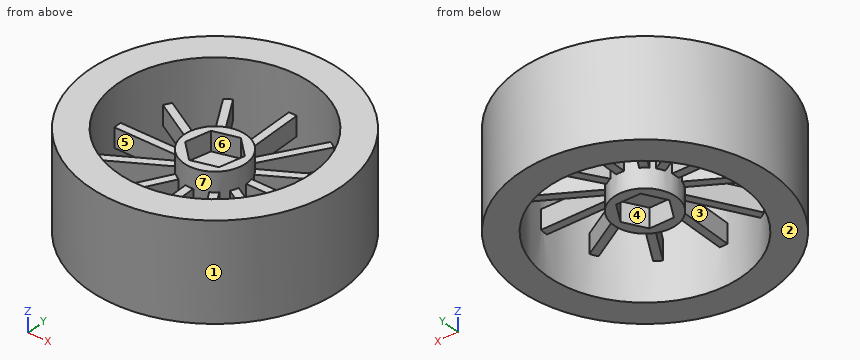
```python
from build123d import *

# Parameters (mm, degrees)
SKETCH_1_R          = 32.5
EXTRUDE_1_DEPTH     = 25
SKETCH_2_R          = 25
CUT_EXTRUDE_1_DEPTH = 25
SKETCH_6_R          = 8
EXTRUDE_3_DEPTH     = 20
SKETCH_7_R          = 8
CUT_EXTRUDE_2_DEPTH = 5
CUT_EXTRUDE_3_DEPTH = 5
CUT_EXTRUDE_4_DEPTH = 5
SKETCH_11_W         = 21
SKETCH_11_H         = 2
EXTRUDE_1_2_DEPTH   = 5
SKETCH_15_W         = 18
SKETCH_15_H         = 2
EXTRUDE_8_DEPTH     = 5
SKETCH_17_W         = 2
SKETCH_17_H         = 19.626417589
EXTRUDE_9_DEPTH     = 5
SKETCH_19_W         = 2
SKETCH_19_H         = 25
EXTRUDE_10_DEPTH    = 5
EXTRUDE_12_DEPTH    = 5
EXTRUDE_13_DEPTH    = 5
EXTRUDE_16_DEPTH    = 5
EXTRUDE_18_DEPTH    = 5
EXTRUDE_20_DEPTH    = 5
EXTRUDE_21_DEPTH    = 5
EXTRUDE_22_DEPTH    = 5
EXTRUDE_23_DEPTH    = 5


with BuildPart() as part:
    # 草图1 → Extrude 1 (new body)
    with BuildSketch(Plane.XY):
        Circle(SKETCH_1_R)
    extrude(amount=EXTRUDE_1_DEPTH)

    # 草图2 → 切除-拉伸1 (cut)
    with BuildSketch(Plane(origin=(0, 0, 0), x_dir=(-1, 0, 0), z_dir=(0, 0, -1))):
        Circle(SKETCH_2_R)
    extrude(amount=-CUT_EXTRUDE_1_DEPTH, mode=Mode.SUBTRACT)



with BuildPart() as body_2:
    # 草图6 → 凸台-拉伸3 (new body)
    with BuildSketch(Plane(origin=(0, 0, 0), x_dir=(-1, 0, 0), z_dir=(0, 0, -1))):
        Circle(SKETCH_6_R)
    extrude(amount=-EXTRUDE_3_DEPTH)

    # 草图7 → 切除-拉伸2 (cut)
    with BuildSketch(Plane(origin=(0, 0, 0), x_dir=(-1, 0, 0), z_dir=(0, 0, -1))):
        Circle(SKETCH_7_R)
    extrude(amount=-CUT_EXTRUDE_2_DEPTH, mode=Mode.SUBTRACT)

    # 草图8 → 切除-拉伸3 (cut)
    with BuildSketch(Plane(origin=(0, 0, 5), x_dir=(-1, 0, 0), z_dir=(0, 0, -1))):
        Polygon((6.204878503, 0), (3.102439251, 5.373582411), (-3.102439251, 5.373582411), (-6.204878503, 0), (-3.102439251, -5.373582411), (3.102439251, -5.373582411), align=None)
    extrude(amount=-CUT_EXTRUDE_3_DEPTH, mode=Mode.SUBTRACT)

    # 草图9 → 切除-拉伸4 (cut)
    with BuildSketch(Plane.XY.offset(20)):
        Polygon((-1.630765345, -6.252377794), (4.599335331, -4.538473114), (6.230100676, 1.713904681), (1.630765345, 6.252377794), (-4.599335331, 4.538473114), (-6.230100676, -1.713904681), align=None)
    extrude(amount=-CUT_EXTRUDE_4_DEPTH, mode=Mode.SUBTRACT)


with BuildPart() as part_1:
    add(part.part)

    add(body_2.part)  # Extrude 1 2 merges body 2
    # 草图11 → Extrude 1 2 (add)
    with BuildSketch(Plane(origin=(0, -0.732123309, 10), x_dir=(-1, 0, 0), z_dir=(0, 0, -1))):
        with Locations((17.554946424, 1)):
            Rectangle(SKETCH_11_W, SKETCH_11_H)
    extrude(amount=-EXTRUDE_1_2_DEPTH)

    # 草图15 → 拉伸-薄壁8 (add)
    with BuildSketch(Plane(origin=(0.783900643, -0.087404702, 10), x_dir=(-1, 0, 0), z_dir=(0, 0, -1))):
        with Locations((-15.204878503, 1)):
            Rectangle(SKETCH_15_W, SKETCH_15_H)
    extrude(amount=-EXTRUDE_8_DEPTH)

    # 草图17 → 拉伸-薄壁9 (add)
    with BuildSketch(Plane(origin=(1.021360023, 0, 10), x_dir=(-1, 0, 0), z_dir=(0, 0, -1))):
        with Locations((1, 15.186791206)):
            Rectangle(SKETCH_17_W, SKETCH_17_H)
    extrude(amount=-EXTRUDE_9_DEPTH)

    # 草图19 → 拉伸-薄壁10 (add)
    with BuildSketch(Plane(origin=(0, 0, 10), x_dir=(-1, 0, 0), z_dir=(0, 0, -1))):
        with Locations((0.222489214, -12.5)):
            Rectangle(SKETCH_19_W, SKETCH_19_H)
    extrude(amount=-EXTRUDE_10_DEPTH)

    # 草图22 → 拉伸-薄壁12 (add)
    with BuildSketch(Plane(origin=(0.523395748, 0, 10), x_dir=(-1, 0, 0), z_dir=(0, 0, -1))):
        Polygon((0, 0), (-13.36975493, 21.124621964), (-11.679785173, 22.194202358), (1.689969757, 1.069580394), align=None)
    extrude(amount=-EXTRUDE_12_DEPTH)

    # 草图23 → 拉伸-薄壁13 (add)
    with BuildSketch(Plane(origin=(0, -0.702264438, 10), x_dir=(-1, 0, 0), z_dir=(0, 0, -1))):
        Polygon((0, 0), (-22.409578035, 12.938175911), (-21.409578035, 14.670226719), (1, 1.732050808), align=None)
    extrude(amount=-EXTRUDE_13_DEPTH)

    # 草图25 → 拉伸-薄壁16 (add)
    with BuildSketch(Plane(origin=(0, 0.899260589, 10), x_dir=(-1, 0, 0), z_dir=(0, 0, -1))):
        Polygon((0, 0), (21.650635095, 12.5), (22.650635095, 10.767949192), (1, -1.732050808), align=None)
    extrude(amount=-EXTRUDE_16_DEPTH)

    # 草图26 → 拉伸-薄壁18 (add)
    with BuildSketch(Plane(origin=(0, 0, 10), x_dir=(-1, 0, 0), z_dir=(0, 0, -1))):
        Polygon((0, 0), (13.491648386, 23.368220483), (15.223699194, 22.368220483), (1.732050808, -1), align=None)
    extrude(amount=-EXTRUDE_18_DEPTH)

    # 草图27 → 拉伸-薄壁20 (add)
    with BuildSketch(Plane(origin=(0, 0, 10), x_dir=(-1, 0, 0), z_dir=(0, 0, -1))):
        Polygon((0, 0), (-23.067411296, -13.317976121), (-24.067411296, -11.585925314), (-1, 1.732050808), align=None)
    extrude(amount=-EXTRUDE_20_DEPTH)

    # 草图28 → 拉伸-薄壁21 (add)
    with BuildSketch(Plane(origin=(0, 0, 10), x_dir=(-1, 0, 0), z_dir=(0, 0, -1))):
        Polygon((0, 0), (-13.731376059, -23.783440992), (-15.463426867, -22.783440992), (-1.732050808, 1), align=None)
    extrude(amount=-EXTRUDE_21_DEPTH)

    # 草图29 → 拉伸-薄壁22 (add)
    with BuildSketch(Plane(origin=(-1.752500167, 0, 10), x_dir=(-1, 0, 0), z_dir=(0, 0, -1))):
        Polygon((0, 0), (13.9695501, -24.195970532), (12.237499292, -25.195970532), (-1.732050808, -1), align=None)
    extrude(amount=-EXTRUDE_22_DEPTH)

    # 草图30 → 拉伸-薄壁23 (add)
    with BuildSketch(Plane.XY.offset(15)):
        Polygon((0, 0), (-22.652441565, -13.078393235), (-23.652441565, -11.346342428), (-1, 1.732050808), align=None)
    extrude(amount=-EXTRUDE_23_DEPTH)


solid = part_1.part
```
Design review of the part built by this model. Coordinates are the model's own, in mm. Face numbers are marked on the shaded views. A direction names the side the tool comes from. Coordinates: 2 decimals unless noted, no trailing zeros. Write each loop counter-clockwise with the first axis right and the second up, starting at its lowest first coordinate (ties: lowest second). Pieces come first, ordered by that corner, then holes.
1) Machinability: for the marked faces 4, 5, 6 and 7, which of the approach directions +Z, -Z, +X, -X, +Y, -Y give a long, thin tool a straight path to every point of the face, cutting with its end or side? Answer none if there is none.
2) Add section C-C (x = -17). Write out the cut boundary in (y, z), plus the area to 3 significant figures.
3) Add section D-D (y = 10.5). Write out the cut boundary in (x, z), plus the area to 3 significant figures.
4) Insertion check: pin 1 (8 mm diameter, centred on x = -14, z = 11.5, fed in from -Y); pin 2 (1.5 mm diameter, centred on x = 2, y = 10.5, fed in from +Z); pin 3 (5 mm diameter, centred on x = -7, y = -8.5, fed in from -Z); pin 4 (11.5 mm diameter, centred on x = 13, y = -7, fed in from +Z). Each pin has a flat end and moves straight along its axis. Give the tip position at first contact, or say it passes through.
5) To check wall thickness, follow L1, parallel to Y at x = 0, z = 9.75; L2, parallel to X at y = 0.5, z = 4.25 (3 decimals); L3, parallel to Y at x = 0, z = 20.25. State the ranges of each line that lie inside material, in increasing order.
6) Add section A-A (z = 7). Write out the cut boundary in (x, y).
7) Add section B-B (y = 24). Write out the cut boundary in (x, z).
8) Mouldability with a two-part tool opening along X and no side actions: class the marked faces 1, 2 and 3 as +X half, -X half, draft (parallel to the pull), parting line (faces both ways), or undercut.
Check result:
1. face 4: -Z
1. face 5: +Z, -Z
1. face 6: +Z
1. face 7: none
2. outline: (-27.7, 0) - (-18.33, 0) - (-18.33, 25) - (-27.7, 25) - close; (-9.81, 10) - (-7.51, 10) - (-7.51, 15) - (-9.81, 15) - close; (-0.73, 10) - (1.27, 10) - (1.27, 15) - (-0.73, 15) - close; (8.4, 10) - (10.71, 10) - (10.71, 15) - (8.4, 15) - close; (18.33, 0) - (27.7, 0) - (27.7, 25) - (18.33, 25) - close
2. area: 502 mm2
3. outline: (-30.76, 0) - (-22.69, 0) - (-22.69, 25) - (-30.76, 25) - close; (-20.63, 10) - (-16.63, 10) - (-16.63, 15) - (-20.63, 15) - close; (-8.37, 10) - (-6.06, 10) - (-6.06, 15) - (-8.37, 15) - close; (-0.98, 10) - (1.02, 10) - (1.02, 15) - (-0.98, 15) - close; (4.8, 10) - (7.17, 10) - (7.17, 15) - (4.8, 15) - close; (15.4, 10) - (19.4, 10) - (19.4, 15) - (15.4, 15) - close; (22.69, 0) - (30.76, 0) - (30.76, 25) - (22.69, 25) - close
3. area: 477 mm2
4. pin 1: stops at y = -30.92
4. pin 2: passes through
4. pin 3: stops at z = 10
4. pin 4: stops at z = 15
5. L1: y = -32.5 to -25, -8 to -5.37, 5.37 to 8, 25 to 32.5
5. L2: x = -32.496 to -24.995, 24.995 to 32.496
5. L3: y = -32.5 to -25, 25 to 32.5
6. outline: circle Ø65 at (0, 0); circle Ø16 at (0, 0); hole circle Ø50 at (0, 0); hole (-6.2, 0) - (-3.1, -5.37) - (3.1, -5.37) - (6.2, 0) - (3.1, 5.37) - (-3.1, 5.37) - close
7. outline: (-21.91, 0) - (-7, 0) - (-7, 25) - (-21.91, 25) - close; (-0.98, 10) - (1.02, 10) - (1.02, 15) - (-0.98, 15) - close; (7, 0) - (21.91, 0) - (21.91, 25) - (7, 25) - close
8. face 1: parting line
8. face 2: draft
8. face 3: undercut
